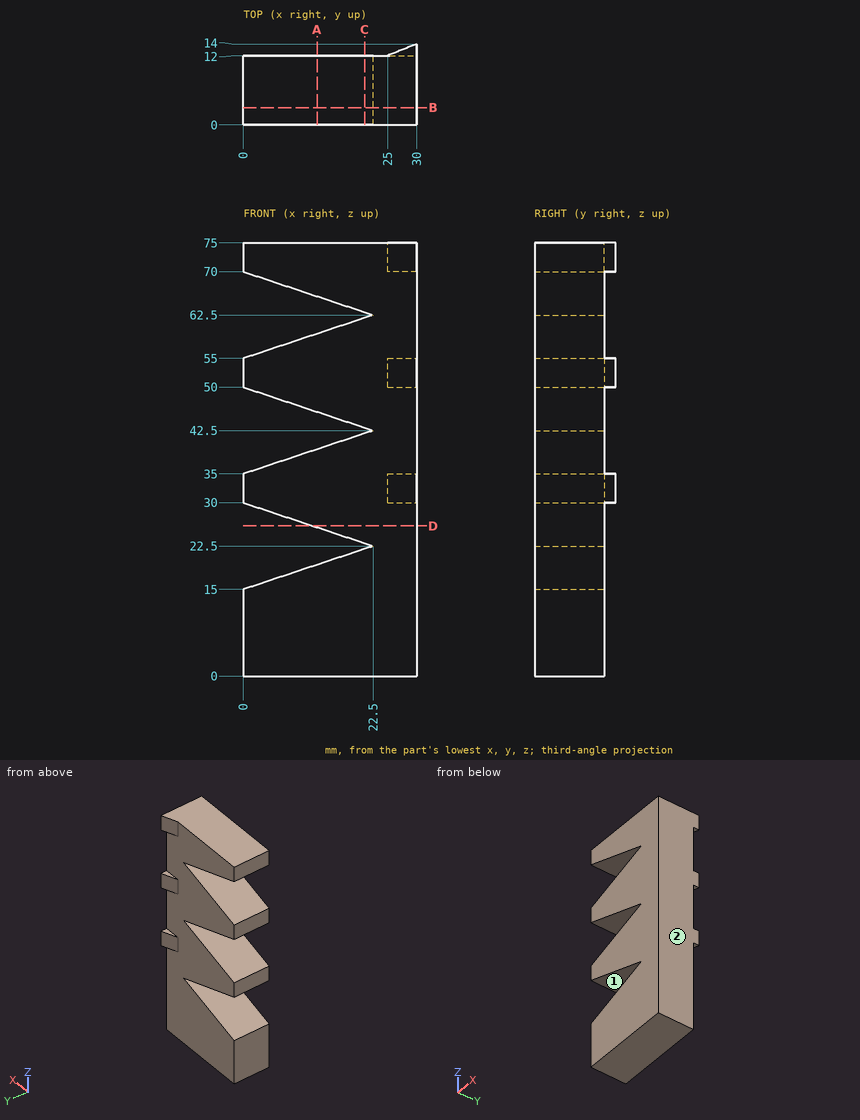
Answer from the drawing. Dimensions are ordinates in mm from the lowest x, y and z of the part. A direction names the side the tool comes from. Give positions to 0.01 mm unless a question says otherwise; leave off trailing zeros. Write each loop counter-clockwise with the first axis right and the second up, starting at its lowest first coordinate (ties: lowest second). Pieces come first, ordered by that corner, then holes. Notation, with made-up numbers: (18.5, -38) - (52.5, -38) arc R36 ccw to (52.5, -2) - close; hole circle Ø6 at (52.5, -23). An arc over 180 degrees is marked (long way). One line per item, written item: value. Start each with the question number.
1. Consider probe 1 along Z at (x, y) = (12.75, 8.5); probe 2 along Z at (x, y) = (3, 1.75); probe 3 along Y at (x, z) = (23.75, 66). Determine where each line is inside the solid, lowest interval first.
2. Find section D-D (z = 26). Write down the section's boundary in (x, y), then the cut area to 3 significant figures.
3. Find section A-A (x = 12.75). Write down the section's boundary in (y, z), then the cut area to 3 significant figures.
4. Given pin 1 (1 mm diameter, centred on x = 27, y = 13, fed in from -Z); pin 2 (1 mm diameter, centred on x = 12.5, z = 23.5, fed in from +Y), each flat-ended and moving along its own axis, determine where each tip first touches the part or whether it passes through.
5. For the marked faces 1 and 2, determine the directions among +Z, -Z, +X, -X, +Y, -Y from which every point of the face is accessible in a straight line to the end or side of a thin tool.
6. Find section B-B (y = 3). Write down the section's boundary in (x, z), then the cut area to 3 significant figures.
7. Find section C-C (x = 21). Write down the section's boundary in (y, z), then the cut area to 3 significant figures.
Geometry results:
1. probe 1: 0 to 19.25, 25.75 to 39.25, 45.75 to 59.25, 65.75 to 75
1. probe 2: 0 to 16, 29 to 36, 49 to 56, 69 to 75
1. probe 3: 0 to 12
2. outline: (12, 0) - (30, 0) - (30, 12) - (12, 12) - close
2. area: 216 mm2
3. outline: (0, 0) - (12, 0) - (12, 19.25) - (0, 19.25) - close; (0, 25.75) - (12, 25.75) - (12, 39.25) - (0, 39.25) - close; (0, 45.75) - (12, 45.75) - (12, 59.25) - (0, 59.25) - close; (0, 65.75) - (12, 65.75) - (12, 75) - (0, 75) - close
3. area: 666 mm2
4. pin 1: z = 30
4. pin 2: through
5. face 1: -X, +Y, -Y
5. face 2: +Z, -Z, +X, +Y, -Y
6. outline: (0, 0) - (30, 0) - (30, 75) - (0, 75) - (0, 70) - (22.5, 62.5) - (0, 55) - (0, 50) - (22.5, 42.5) - (0, 35) - (0, 30) - (22.5, 22.5) - (0, 15) - close
6. area: 1,740 mm2
7. outline: (0, 0) - (12, 0) - (12, 22) - (0, 22) - close; (0, 23) - (12, 23) - (12, 42) - (0, 42) - close; (0, 43) - (12, 43) - (12, 62) - (0, 62) - close; (0, 63) - (12, 63) - (12, 75) - (0, 75) - close
7. area: 864 mm2
